The model under review builds one solid part; all positions refer to its coordinate system, in mm. Give positions to 0.01 mm unless a question says otherwise; leave off trailing zeros. Order: outer loops, then holes, each group sorted by start corner. A loop starts at its lowest first (then second) coordinate and runs counter-clockwise, first axis right, second up. Notation, with made-up numbers: (69, 72.5) - (95, 72.5) arc R16 cw to (95, 101.5) - close; hole circle Ø7 at (73.5, -30.75). An arc over 180 degrees is marked (long way). Use CSV: the item, a comma, the result in double quotes. Start each with the question number.
1. Take a section at B-B, the plane y = 23.5. State the section outline as (x, z) points.
2. For pin 1 (0.8 mm diameter, centred on x = -7, z = 1, fed in from +Y); pin 2 (0.8 mm diameter, centred on x = -11, z = 0.5, fed in from +Y); pin 3 (0.8 mm diameter, centred on x = -0.5, z = 1, fed in from +Y), all flat-tipped, find the tip position at first contact; note any pin that passes through.
3. Take a section at A-A, the plane x = -18.5. State the section outline as (y, z) points, then the cut area to 4 significant figures.
4. To check wall thickness, follow line 1 (Y direction, x = -17.25, z = 1.05); line 2 (X direction, y = 24, z = 0.55); line 3 (X direction, y = 30.5, z = 1.25). State the ranges of each line that lie inside material, in increasing order. Write a range as [from, to].
5. Take a section at D-D, the plane z = 0.5. Count the separate pieces of the cut face and the enclosed holes in it, then the cut area to 3 significant figures.
6. Take a section at C-C, the plane y = 33.5. State the section outline as (x, z) points.
```python
from build123d import *

# Parameters (mm, degrees)
BOSS_EXTRUDE1_DEPTH = 1.5


with BuildPart() as part:
    # Sketch1 → Boss-Extrude1 (new body)
    with BuildSketch(Plane.XY):
        with BuildLine():
            Line((-19, 0), (0, 0))
            Line((0, 0), (0, 7))
            Line((0, 7), (-2, 7))
            ThreePointArc((-2, 7), (-2.707106781, 7.292893219), (-3, 8))
            Line((-3, 8), (-3, 24))
            ThreePointArc((-3, 24), (-2.707106781, 24.707106781), (-2, 25))
            Line((-2, 25), (0, 25))
            Line((0, 25), (0, 35.5))
            Line((0, 35.5), (-2, 35.5))
            Line((-2, 35.5), (-2, 40.5))
            Line((-2, 40.5), (-9.5, 40.5))
            ThreePointArc((-9.5, 40.5), (-12.328427125, 41.671572875), (-13.5, 44.5))
            Line((-13.5, 44.5), (-30, 44.5))
            Line((-30, 44.5), (-30, 16))
            ThreePointArc((-30, 16), (-29.012989214, 12.12927861), (-26.292993631, 9.203821656))
            ThreePointArc((-26.292993631, 9.203821656), (-24.610522135, 7.394260653), (-24, 5))
            ThreePointArc((-24, 5), (-22.535533906, 1.464466094), (-19, 0))
        make_face()
        with BuildLine():
            Line((-25, 35.5), (-25, 18.5))
            ThreePointArc((-25, 18.5), (-24, 17.5), (-23, 18.5))
            Line((-23, 18.5), (-23, 35.5))
            ThreePointArc((-23, 35.5), (-24, 36.5), (-25, 35.5))
        make_face(mode=Mode.SUBTRACT)
        with BuildLine():
            Line((-7.5, 5), (-7.5, 27))
            ThreePointArc((-7.5, 27), (-8.085786438, 28.414213562), (-9.5, 29))
            Line((-9.5, 29), (-13.5, 29))
            ThreePointArc((-13.5, 29), (-14.914213562, 28.414213562), (-15.5, 27))
            Line((-15.5, 27), (-15.5, 21.5))
            Line((-15.5, 21.5), (-19, 21.5))
            ThreePointArc((-19, 21.5), (-20.414213562, 20.914213562), (-21, 19.5))
            Line((-21, 19.5), (-21, 12.5))
            ThreePointArc((-21, 12.5), (-20.414213562, 11.085786438), (-19, 10.5))
            Line((-19, 10.5), (-15.5, 10.5))
            Line((-15.5, 10.5), (-15.5, 5))
            ThreePointArc((-15.5, 5), (-14.914213562, 3.585786438), (-13.5, 3))
            Line((-13.5, 3), (-9.5, 3))
            ThreePointArc((-9.5, 3), (-8.085786438, 3.585786438), (-7.5, 5))
        make_face(mode=Mode.SUBTRACT)
    extrude(amount=BOSS_EXTRUDE1_DEPTH)


solid = part.part
```
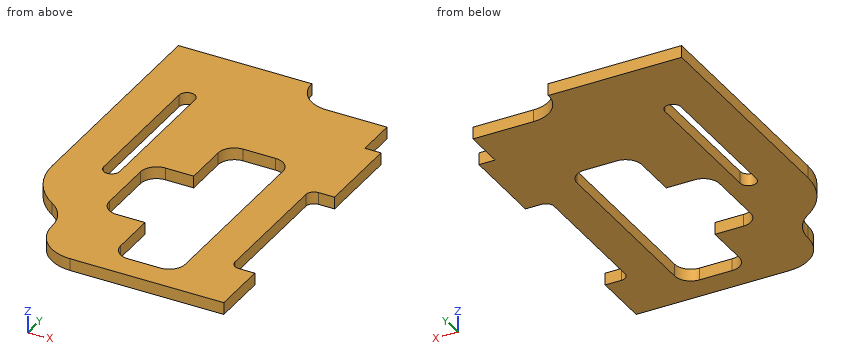
Determined:
1,outline,"(-30, 0) - (-25, 0) - (-25, 1.5) - (-30, 1.5) - close; (-23, 0) - (-15.5, 0) - (-15.5, 1.5) - (-23, 1.5) - close; (-7.5, 0) - (-3, 0) - (-3, 1.5) - (-7.5, 1.5) - close"
2,pin 1,"stops at y = 40.5"
2,pin 2,"stops at y = 40.98"
2,pin 3,"stops at y = 35.5"
3,outline,"(0, 0) - (10.5, 0) - (10.5, 1.5) - (0, 1.5) - close; (21.5, 0) - (44.5, 0) - (44.5, 1.5) - (21.5, 1.5) - close"
3,area,"50.25 mm²"
4,line 1,"y = [0, 10.5], [21.5, 44.5]"
4,line 2,"x = [-30, -25], [-23, -15.5], [-7.5, -3]"
4,line 3,"x = [-30, -25], [-23, 0]"
5,separate pieces,"1"
5,enclosed holes,"2"
5,area,"855 mm²"
6,outline,"(-30, 0) - (-25, 0) - (-25, 1.5) - (-30, 1.5) - close; (-23, 0) - (0, 0) - (0, 1.5) - (-23, 1.5) - close"
